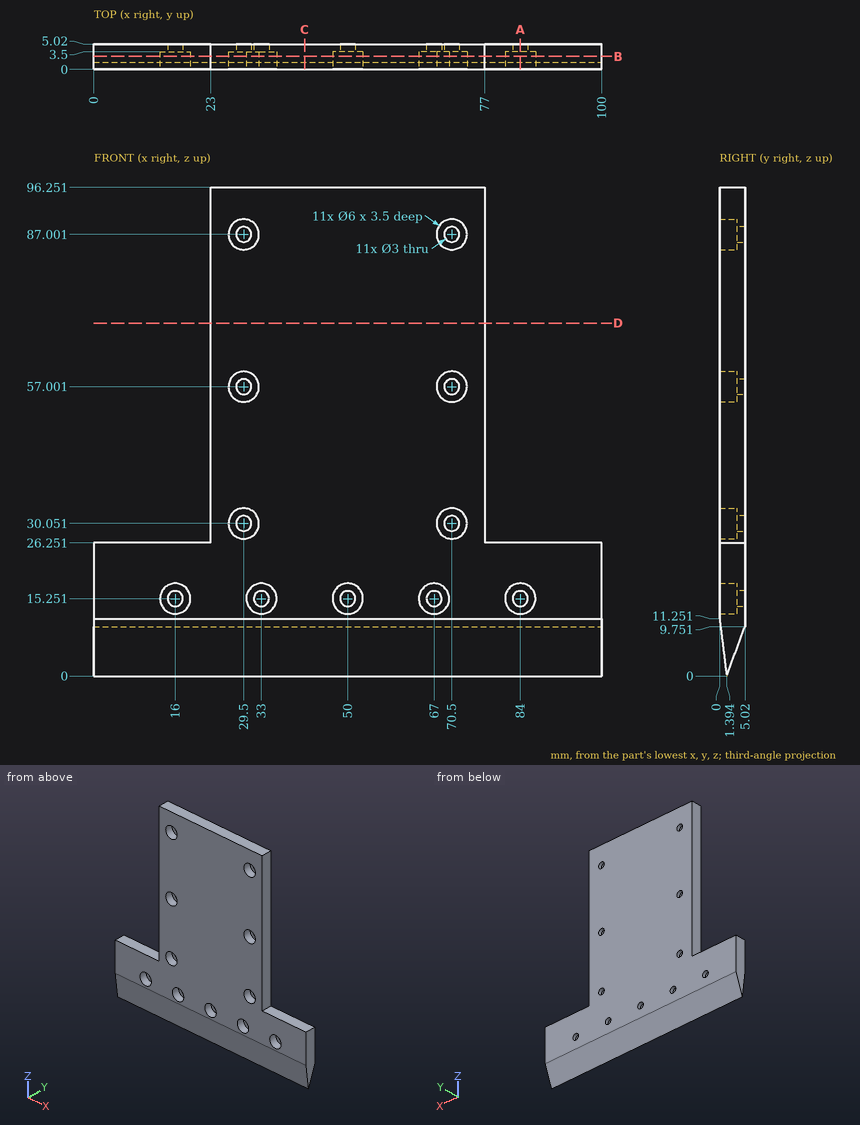
Geometry check sheet. Reference: drawing and pictorial views, mm from the part's lowest x, y, z. Round coordinates to 2 decimals unless told otherwise and drop trailing zeros. Order: outer loops, then holes, each group sorted by start corner. A loop starts at its lowest first (then second) coordinate and runs counter-clockwise, first axis right, second up. Notation, with made-up numbers: (79, 26) - (110, 26) arc R24 cw to (110, 40) - close; hole circle Ø7 at (42, 28.25). An arc over 180 degrees is marked (long way). Use a Markdown table: item, result. Add a question column.
1) Section check A-A (x = 84). Record the cut outline in (y, z).
2) Section check C-C (x = 41.5). Record the cut outline in (y, z), then the cut area to 3 significant figures.
3) Gauge pin test, flat end, axial feed: P1, Ø1.8, axis at x = 67, z = 14.5, coming from the -Y side. Record the tip position at first contact, or that the pin passes through.
4) Section check D-D (z = 69.5). Record the cut outline in (x, y).
5) Section check B-B (y = 2.6). Count the separate pieces of the cut face and the enclosed holes in it, then the cut area to 3 significant figures.
6) Thickness scan on line 1 along X through (y, z) = (1.1, 56.5); line 2 along X through (y, z) = (2.35, 15); line 3 along X through (y, z) = (0.5, 36.5). Record the ranges inside material, lowest first.
Established:
| question | item | result |
|---|---|---|
| 1 | outline | (0, 11.25) - (1.39, 0) - (5.02, 9.75) - (5.02, 13.75) - (3.5, 13.75) - (3.5, 12.25) - (0, 12.25) - close; (0, 18.25) - (3.5, 18.25) - (3.5, 16.75) - (5.02, 16.75) - (5.02, 26.25) - (0, 26.25) - close |
| 2 | outline | (0, 11.25) - (1.39, 0) - (5.02, 9.75) - (5.02, 96.25) - (0, 96.25) - close |
| 2 | area | 458 mm2 |
| 3 | P1 | y = 3.5 |
| 4 | outline | (23, 0) - (77, 0) - (77, 5.02) - (23, 5.02) - close |
| 5 | separate pieces | 1 |
| 5 | enclosed holes | 11 |
| 5 | area | 5,770 mm2 |
| 6 | line 1 | 23 to 26.54, 32.46 to 67.54, 73.46 to 77 |
| 6 | line 2 | 0 to 13.01, 18.99 to 30.01, 35.99 to 47.01, 52.99 to 64.01, 69.99 to 81.01, 86.99 to 100 |
| 6 | line 3 | 23 to 77 |
